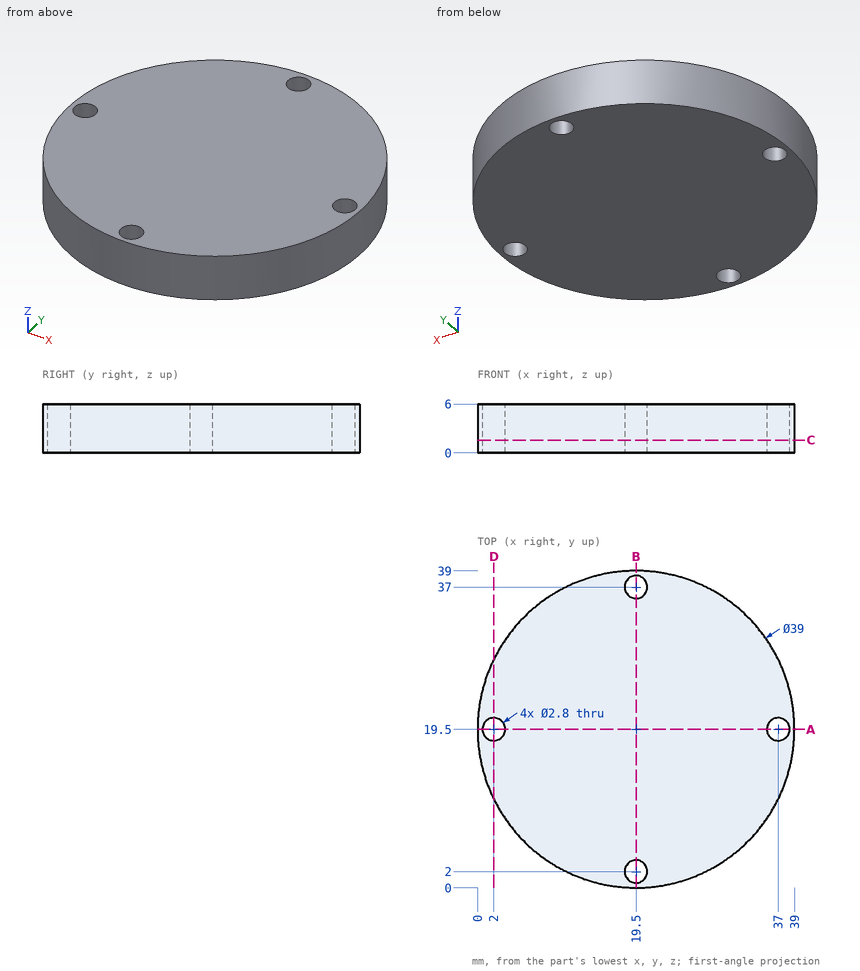
Verification items for this drawing (mm, ordinates from the low corner). Coordinates: 2 decimals unless noted, no trailing zeros. Loops run counter-clockwise (first coordinate to the right, second up) from the corner with the lowest first, then second, coordinate; pieces in that order, holes last. Notation, with made-up numbers: (-24, -6) -> (31, -6) arc R22 ccw to (31, 23) -> close; hole circle Ø4 at (-5.5, 13). An arc over 180 degrees is marked (long way). Answer in a Markdown table with one row per item. Add a question column.
1. Material ranges on probe 1 along Y at (x, z) = (19.5, 4); probe 2 along Y at (x, z) = (3, 3); probe 3 along Y at (x, z) = (2, 3.6), recorded low to high. Write a range as [from, to].
2. Depth check by flat-ended pin: P1, Ø2, axis at x = 24.5, z = 4, coming from the -Y side; P2, Ø1, axis at y = 4.5, z = 4.5, coming from the +X side. Enter the tip coordinate at first touch or a pass-through.
3. Section check C-C, the plane z = 1.55. Enter the section's corners in (x, y), then the cut area to 3 significant figures.
4. Section check D-D, the plane x = 2. Enter the section's corners in (y, z), then the cut area to 3 significant figures.
5. Section check A-A, the plane y = 19.5. Enter the section's corners in (x, z).
Derived:
| question | item | result |
|---|---|---|
| 1 | probe 1 | y = [0, 0.6], [3.4, 35.6], [38.4, 39] |
| 1 | probe 2 | y = [9.11, 18.52], [20.48, 29.89] |
| 1 | probe 3 | y = [10.9, 18.1], [20.9, 28.1] |
| 2 | P1 | stops at y = 0.41 |
| 2 | P2 | stops at x = 32.54 |
| 3 | outline | circle Ø39 at (19.5, 19.5); hole circle Ø2.8 at (2, 19.5); hole circle Ø2.8 at (19.5, 2); hole circle Ø2.8 at (19.5, 37); hole circle Ø2.8 at (37, 19.5) |
| 3 | area | 1,170 mm² |
| 4 | outline | (10.9, 0) -> (18.1, 0) -> (18.1, 6) -> (10.9, 6) -> close; (20.9, 0) -> (28.1, 0) -> (28.1, 6) -> (20.9, 6) -> close |
| 4 | area | 86.4 mm² |
| 5 | outline | (0, 0) -> (0.6, 0) -> (0.6, 6) -> (0, 6) -> close; (3.4, 0) -> (35.6, 0) -> (35.6, 6) -> (3.4, 6) -> close; (38.4, 0) -> (39, 0) -> (39, 6) -> (38.4, 6) -> close |
